Verification items for the finished model (mm, model axes). Face numbers are marked on the shaded views. A direction names the side the tool comes from. Coordinates: 2 decimals unless noted, no trailing zeros. Write each loop counter-clockwise with the first axis right and the second up, starting at its lowest first coordinate (ties: lowest second). Pieces come first, ordered by that corner, then holes. Notation, with made-up numbers: (79.25, -3) - (98.25, -3) arc R20 cw to (98.25, 36) - close; hole circle Ø4 at (28.5, -19). An arc over 180 degrees is marked (long way). Use one line per item in the form item = value. Start each with the question number.
(1) Sectioned sample at D-D (z = 1.25). Record the cut outline in (x, y) (3 decimals).
(2) Tool access check on the marked faces 1, 2, 3, 4 and 5. Record the directions out of +Z, -Z, +X, -X, +Y, -Y that give a thin tool (end or side, any length) a straight path to the whole face; none if there is none.
(3) Material ranges on line 1 (Y direction, x = 0, z = 1.3) (3 decimals); line 2 (Z direction, x = -5.25, y = 2.5); line 3 (X direction, y = 0, z = -5.75) (3 decimals), recorded low to high. Write a range as [from, to].
(4) Sectioned sample at C-C (y = -9). Record the cut outline in (x, z), and give its area (3 significant figures).
(5) Sectioned sample at A-A (y = 0). Record the cut outline in (x, z) (3 decimals), and give its area (3 significant figures).
(6) Mould release check, pull along Z, two halves, no side actions. Record for the marked faces 6, 7 and 8: released by +Z, released by -Z, zero draft, split by the parting line, or undercut.
(7) Gauge pin test, flat ends, axial feed: pin 1 Ø2 at (x, z) = (-4.5, -10.5) entering from -Y; pin 2 Ø5 at (x, z) = (5, -10) entering from -Y; pin 3 Ø2 at (y, z) = (0.5, -10.5) entering from +X (3 decimals). Record the tip position at first contact, or that the pin passes through.
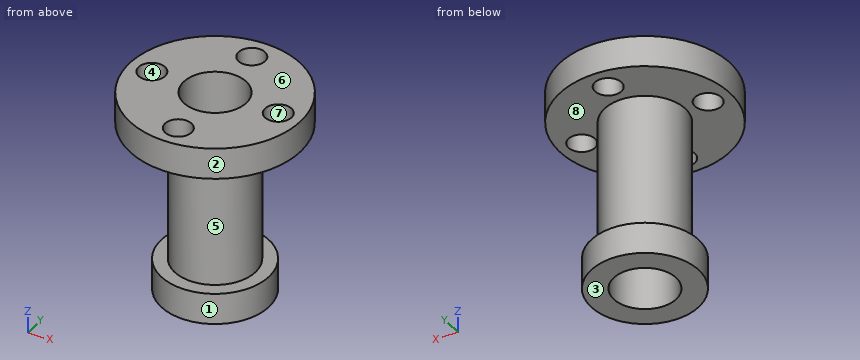
from build123d import *

# Parameters (mm, degrees)
F0_R     = 10.925
F0_R_2   = 4
F1_DEPTH = 4
F2_R     = 1.7
F3_DEPTH = 4
F4_R     = 5.175
F4_R_2   = 4
F5_DEPTH = 11
F6_DEPTH = 11
F7_R     = 6.9
F7_R_2   = 5.175
F8_DEPTH = 4


with BuildPart() as f1:
    # F0 (on Top) → F1 (new body)
    with BuildSketch(Plane.XY):
        Circle(F0_R)
        Circle(F0_R_2, mode=Mode.SUBTRACT)
    extrude(amount=F1_DEPTH)

    # F2 (on face) → F3 (cut, through all)
    with BuildSketch(Plane.XY.offset(4)):
        with Locations((0, 8)):
            Circle(F2_R)
        with Locations((-8, 0)):
            Circle(F2_R)
        with Locations((8, 0)):
            Circle(F2_R)
        with Locations((0, -8)):
            Circle(F2_R)
    extrude(amount=-F3_DEPTH, mode=Mode.SUBTRACT)

    # F4 (on face) → F5 (join)
    with BuildSketch(Plane(origin=(0, 0, 0), x_dir=(1, 0, 0), z_dir=(0, 0, -1))):
        Circle(F4_R)
        Circle(F4_R_2, mode=Mode.SUBTRACT)
    extrude(amount=F5_DEPTH)

    # F6 (add): a face of the model
    f6_faces = [f1.faces().sort_by_distance(p)[0] for p in [
        (-5.0286288963, 0, -11),
    ]]
    extrude(f6_faces, amount=F6_DEPTH)

    # F7 (on face) → F8 (join)
    with BuildSketch(Plane(origin=(0, 0, -22), x_dir=(1, 0, 0), z_dir=(0, 0, -1))):
        Circle(F7_R)
        Circle(F7_R_2, mode=Mode.SUBTRACT)
    extrude(amount=-F8_DEPTH)


solid = f1.part
Answers below:
q1.outline = circle Ø21.85 at (0, 0); hole circle Ø3.4 at (-8, 0); hole circle Ø8 at (0, 0); hole circle Ø3.4 at (0, -8); hole circle Ø3.4 at (0, 8); hole circle Ø3.4 at (8, 0)
q2.face_1 = -Z
q2.face_2 = +Z, -Z
q2.face_3 = -Z, +X, -X, +Y, -Y
q2.face_4 = +Z
q2.face_5 = none
q3.line_1 = [-10.925, -9.7], [-6.3, -4], [4, 6.3], [9.7, 10.925]
q3.line_2 = [-22, -18], [0, 4]
q3.line_3 = [-5.175, -4], [4, 5.175]
q4.outline = (-6.19, 0) - (-1.37, 0) - (-1.37, 4) - (-6.19, 4) - close; (1.37, 0) - (6.19, 0) - (6.19, 4) - (1.37, 4) - close
q4.area = 38.5 mm2
q5.outline = (-10.925, 0) - (-9.7, 0) - (-9.7, 4) - (-10.925, 4) - close; (-6.9, -22) - (-4, -22) - (-4, 4) - (-6.3, 4) - (-6.3, 0) - (-5.175, 0) - (-5.175, -18) - (-6.9, -18) - close; (4, -22) - (6.9, -22) - (6.9, -18) - (5.175, -18) - (5.175, 0) - (6.3, 0) - (6.3, 4) - (4, 4) - close; (9.7, 0) - (10.925, 0) - (10.925, 4) - (9.7, 4) - close
q5.area = 93.7 mm2
q6.face_6 = released by +Z
q6.face_7 = zero draft
q6.face_8 = undercut
q7.pin_1 = -3.81
q7.pin_2 = -4.53
q7.pin_3 = 5.175
